Geometry check sheet. Reference: the model listing, model coordinates, mm. A direction names the side the tool comes from. Round coordinates to 2 decimals unless told otherwise and drop trailing zeros. Loops run counter-clockwise (first coordinate to the right, second up) from the corner with the lowest first, then second, coordinate; pieces in that order, holes last. Notation, with made-up numbers: (-39, -8.5) -> (16, -8.5) arc R28 cw to (16, 21.5) -> close; hole circle Ø7 at (-26, 69). An arc over 180 degrees is marked (long way). Use a Markdown table: item, result. Add a question column.
Q1. Gauge pin test, flat ends, axial feed: P1, Ø1.5, axis at x = 14.5, y = 34, coming from the -Z side; P2, Ø0.8, axis at x = 14, z = 1.5, coming from the +Y side. Record the tip position at first contact, or that the pin passes through.
Q2. Material ranges on L1, parallel to X at y = 70.5, z = 2.8 (3 decimals); L2, parallel to Z at x = 10, y = 39 (3 decimals); L3, parallel to Y at x = 93.5, z = 0.45, recorded low to high.
Q3. Release check for a two-part mould opening along X. For faces 4 (the face through (50, 39, -0.178)), 5 (the face through (101.778, 38, 2)), 6 (the face through (-0.178, 39, 2)), 7 (the face through (101.6, 39, 2)) record: released by +X, released by -X, zero draft, split by the parting line, or undercut.
Q4. Sectioned sample at C-C, the plane y = 13.5. Enter the section's corners in (x, z) (3 decimals), then the cut area to 3 significant figures.
Q5. Set-up check for faces 1 (the face through (88.9, 45, 2)), 2 (the face through (6, 76.378, 2)), 3 (the face through (12.878, 45, 2)): record each of +Z, -Z, +X, -X, +Y, -Y from which the full face is reachable in a straight line by a thin tool's end or side.
Q6. Sectioned sample at A-A, the plane y = 52. Enter the section's corners in (x, z) (3 decimals).
Q7. Sectioned sample at B-B, the plane x = 14. Enter the section's corners in (y, z) (3 decimals).
```python
from build123d import *

# Parameters (mm, degrees)
BOSS_EXTRUDE1_DEPTH = 3.175
FILLET5_R           = 1.27
SHELL2_START        = -0.1778
SHELL2_OUTLINE_W    = 75.8444
SHELL2_OUTLINE_H    = 3.5306
SHELL2_DEPTH        = 0.1778
SHELL2_START_2      = 14.942805851
SHELL2_2_OUTLINE_W  = 2.8194
SHELL2_2_OUTLINE_H  = 3.5306
SHELL2_2_DEPTH      = 0.1778
SHELL2_3_DEPTH      = 3.175
SHELL2_4_DEPTH      = 0.1778
SHELL2_START_3      = 3.175
SHELL2_5_DEPTH      = 0.1778
SHELL2_6_DEPTH      = 3.5306


with BuildPart() as part:
    # Sketch1 → Boss-Extrude1 (new body)
    with BuildSketch(Plane.XY):
        Polygon((50.8, 0), (50.8, 76.2), (15.875, 76.2), (15.875, 14.942805851), (12.7, 14.942805851), (12.7, 76.2), (0, 76.2), (0, 0), align=None)
        Polygon((85.725, 76.2), (50.8, 76.2), (50.8, 0), (101.6, 0), (101.6, 76.2), (88.9, 76.2), (88.9, 14.942805851), (85.725, 14.942805851), align=None)
    extrude(amount=BOSS_EXTRUDE1_DEPTH)

    # Fillet5
    fillet5_edges = [part.edges().sort_by_distance(p)[0] for p in [
        (0, 0, 1.5875),
        (0, 76.2, 1.5875),
        (12.7, 76.2, 1.5875),
        (15.875, 76.2, 1.5875),
        (85.725, 76.2, 1.5875),
        (88.9, 76.2, 1.5875),
        (101.6, 76.2, 1.5875),
        (101.6, 0, 1.5875),
    ]]
    fillet(fillet5_edges, radius=FILLET5_R)

    # Shell2: read off the stored shape, not the designer's step
    # Shell2 outline → Shell2 (add)
    with BuildSketch(Plane(origin=(0, 0, 0), x_dir=(1, 0, 0), z_dir=(0, 1, 0)).offset(SHELL2_START)):
        with Locations((50.8, -1.5875)):
            Rectangle(SHELL2_OUTLINE_W, SHELL2_OUTLINE_H)
    extrude(amount=SHELL2_DEPTH)

    # Shell2 2 outline → Shell2 2 (add)
    with BuildSketch(Plane(origin=(0, 0, 0), x_dir=(1, 0, 0), z_dir=(0, 1, 0)).offset(SHELL2_START_2)):
        with Locations((87.3125, -1.5875)):
            Rectangle(SHELL2_2_OUTLINE_W, SHELL2_2_OUTLINE_H)
        with Locations((14.2875, -1.5875)):
            Rectangle(SHELL2_2_OUTLINE_W, SHELL2_2_OUTLINE_H)
    extrude(amount=SHELL2_2_DEPTH)

    # Shell2 3 outline → Shell2 3 (cut)
    with BuildSketch(Plane.XY):
        with BuildLine():
            Line((1.27, 0), (100.33, 0))
            ThreePointArc((100.33, 0), (101.228025612, 0.371974388), (101.6, 1.27))
            Line((101.6, 1.27), (101.6, 74.93))
            ThreePointArc((101.6, 74.93), (101.228025612, 75.828025612), (100.33, 76.2))
            Line((100.33, 76.2), (90.17, 76.2))
            ThreePointArc((90.17, 76.2), (89.271974388, 75.828025612), (88.9, 74.93))
            Line((88.9, 74.93), (88.9, 14.942805851))
            Line((88.9, 14.942805851), (85.725, 14.942805851))
            Line((85.725, 14.942805851), (85.725, 74.93))
            ThreePointArc((85.725, 74.93), (85.353025612, 75.828025612), (84.455, 76.2))
            Line((84.455, 76.2), (17.145, 76.2))
            ThreePointArc((17.145, 76.2), (16.246974388, 75.828025612), (15.875, 74.93))
            Line((15.875, 74.93), (15.875, 14.942805851))
            Line((15.875, 14.942805851), (12.7, 14.942805851))
            Line((12.7, 14.942805851), (12.7, 74.93))
            ThreePointArc((12.7, 74.93), (12.328025612, 75.828025612), (11.43, 76.2))
            Line((11.43, 76.2), (1.27, 76.2))
            ThreePointArc((1.27, 76.2), (0.371974388, 75.828025612), (0, 74.93))
            Line((0, 74.93), (0, 1.27))
            ThreePointArc((0, 1.27), (0.371974388, 0.371974388), (1.27, 0))
        make_face()
    extrude(amount=SHELL2_3_DEPTH, mode=Mode.SUBTRACT)

    # Shell2 4 outline → Shell2 4 (add)
    with BuildSketch(Plane.XY.offset(SHELL2_START)):
        with BuildLine():
            Line((88.7222, -0.1778), (100.33, -0.1778))
            ThreePointArc((100.33, -0.1778), (101.353749198, 0.246250802), (101.7778, 1.27))
            Line((101.7778, 1.27), (101.7778, 74.93))
            ThreePointArc((101.7778, 74.93), (101.353749198, 75.953749198), (100.33, 76.3778))
            Line((100.33, 76.3778), (90.17, 76.3778))
            ThreePointArc((90.17, 76.3778), (89.146250802, 75.953749198), (88.7222, 74.93))
            Line((88.7222, 74.93), (88.7222, 14.942805851))
            Line((88.7222, 14.942805851), (85.9028, 14.942805851))
            Line((85.9028, 14.942805851), (85.9028, 74.93))
            ThreePointArc((85.9028, 74.93), (85.478749198, 75.953749198), (84.455, 76.3778))
            Line((84.455, 76.3778), (17.145, 76.3778))
            ThreePointArc((17.145, 76.3778), (16.121250802, 75.953749198), (15.6972, 74.93))
            Line((15.6972, 74.93), (15.6972, 14.942805851))
            Line((15.6972, 14.942805851), (12.8778, 14.942805851))
            Line((12.8778, 14.942805851), (12.8778, 74.93))
            ThreePointArc((12.8778, 74.93), (12.453749198, 75.953749198), (11.43, 76.3778))
            Line((11.43, 76.3778), (1.27, 76.3778))
            ThreePointArc((1.27, 76.3778), (0.246250802, 75.953749198), (-0.1778, 74.93))
            Line((-0.1778, 74.93), (-0.1778, 1.27))
            ThreePointArc((-0.1778, 1.27), (0.246250802, 0.246250802), (1.27, -0.1778))
            Line((1.27, -0.1778), (12.8778, -0.1778))
            Line((12.8778, -0.1778), (12.8778, 0))
            Line((12.8778, 0), (88.7222, 0))
            Line((88.7222, 0), (88.7222, -0.1778))
        make_face()
    extrude(amount=SHELL2_4_DEPTH)

    # Shell2 5 outline → Shell2 5 (add)
    with BuildSketch(Plane.XY.offset(SHELL2_START_3)):
        with BuildLine():
            Line((88.7222, -0.1778), (100.33, -0.1778))
            ThreePointArc((100.33, -0.1778), (101.353749198, 0.246250802), (101.7778, 1.27))
            Line((101.7778, 1.27), (101.7778, 74.93))
            ThreePointArc((101.7778, 74.93), (101.353749198, 75.953749198), (100.33, 76.3778))
            Line((100.33, 76.3778), (90.17, 76.3778))
            ThreePointArc((90.17, 76.3778), (89.146250802, 75.953749198), (88.7222, 74.93))
            Line((88.7222, 74.93), (88.7222, 14.942805851))
            Line((88.7222, 14.942805851), (85.9028, 14.942805851))
            Line((85.9028, 14.942805851), (85.9028, 74.93))
            ThreePointArc((85.9028, 74.93), (85.478749198, 75.953749198), (84.455, 76.3778))
            Line((84.455, 76.3778), (17.145, 76.3778))
            ThreePointArc((17.145, 76.3778), (16.121250802, 75.953749198), (15.6972, 74.93))
            Line((15.6972, 74.93), (15.6972, 14.942805851))
            Line((15.6972, 14.942805851), (12.8778, 14.942805851))
            Line((12.8778, 14.942805851), (12.8778, 74.93))
            ThreePointArc((12.8778, 74.93), (12.453749198, 75.953749198), (11.43, 76.3778))
            Line((11.43, 76.3778), (1.27, 76.3778))
            ThreePointArc((1.27, 76.3778), (0.246250802, 75.953749198), (-0.1778, 74.93))
            Line((-0.1778, 74.93), (-0.1778, 1.27))
            ThreePointArc((-0.1778, 1.27), (0.246250802, 0.246250802), (1.27, -0.1778))
            Line((1.27, -0.1778), (12.8778, -0.1778))
            Line((12.8778, -0.1778), (12.8778, 0))
            Line((12.8778, 0), (88.7222, 0))
            Line((88.7222, 0), (88.7222, -0.1778))
        make_face()
    extrude(amount=SHELL2_5_DEPTH)

    # Shell2 6 outline → Shell2 6 (add)
    with BuildSketch(Plane.XY.offset(SHELL2_START)):
        with BuildLine():
            Line((88.7222, -0.1778), (100.33, -0.1778))
            ThreePointArc((100.33, -0.1778), (101.353749198, 0.246250802), (101.7778, 1.27))
            Line((101.7778, 1.27), (101.7778, 74.93))
            ThreePointArc((101.7778, 74.93), (101.353749198, 75.953749198), (100.33, 76.3778))
            Line((100.33, 76.3778), (90.17, 76.3778))
            ThreePointArc((90.17, 76.3778), (89.146250802, 75.953749198), (88.7222, 74.93))
            Line((88.7222, 74.93), (88.7222, 14.942805851))
            Line((88.7222, 14.942805851), (88.9, 14.942805851))
            Line((88.9, 14.942805851), (88.9, 74.93))
            ThreePointArc((88.9, 74.93), (89.271974388, 75.828025612), (90.17, 76.2))
            Line((90.17, 76.2), (100.33, 76.2))
            ThreePointArc((100.33, 76.2), (101.228025612, 75.828025612), (101.6, 74.93))
            Line((101.6, 74.93), (101.6, 1.27))
            ThreePointArc((101.6, 1.27), (101.228025612, 0.371974388), (100.33, 0))
            Line((100.33, 0), (88.7222, 0))
            Line((88.7222, 0), (88.7222, -0.1778))
        make_face()
        with BuildLine():
            Line((1.27, -0.1778), (12.8778, -0.1778))
            Line((12.8778, -0.1778), (12.8778, 0))
            Line((12.8778, 0), (1.27, 0))
            ThreePointArc((1.27, 0), (0.371974388, 0.371974388), (0, 1.27))
            Line((0, 1.27), (0, 74.93))
            ThreePointArc((0, 74.93), (0.371974388, 75.828025612), (1.27, 76.2))
            Line((1.27, 76.2), (11.43, 76.2))
            ThreePointArc((11.43, 76.2), (12.328025612, 75.828025612), (12.7, 74.93))
            Line((12.7, 74.93), (12.7, 14.942805851))
            Line((12.7, 14.942805851), (12.8778, 14.942805851))
            Line((12.8778, 14.942805851), (12.8778, 74.93))
            ThreePointArc((12.8778, 74.93), (12.453749198, 75.953749198), (11.43, 76.3778))
            Line((11.43, 76.3778), (1.27, 76.3778))
            ThreePointArc((1.27, 76.3778), (0.246250802, 75.953749198), (-0.1778, 74.93))
            Line((-0.1778, 74.93), (-0.1778, 1.27))
            ThreePointArc((-0.1778, 1.27), (0.246250802, 0.246250802), (1.27, -0.1778))
        make_face()
        with BuildLine():
            Line((85.725, 14.942805851), (85.9028, 14.942805851))
            Line((85.9028, 14.942805851), (85.9028, 74.93))
            ThreePointArc((85.9028, 74.93), (85.478749198, 75.953749198), (84.455, 76.3778))
            Line((84.455, 76.3778), (17.145, 76.3778))
            ThreePointArc((17.145, 76.3778), (16.121250802, 75.953749198), (15.6972, 74.93))
            Line((15.6972, 74.93), (15.6972, 14.942805851))
            Line((15.6972, 14.942805851), (15.875, 14.942805851))
            Line((15.875, 14.942805851), (15.875, 74.93))
            ThreePointArc((15.875, 74.93), (16.246974388, 75.828025612), (17.145, 76.2))
            Line((17.145, 76.2), (84.455, 76.2))
            ThreePointArc((84.455, 76.2), (85.353025612, 75.828025612), (85.725, 74.93))
            Line((85.725, 74.93), (85.725, 14.942805851))
        make_face()
    extrude(amount=SHELL2_6_DEPTH)


solid = part.part
```
Values:
| question | item | result |
|---|---|---|
| 1 | P1 | through |
| 1 | P2 | y = 15.12 |
| 2 | L1 | -0.178 to 0, 12.7 to 12.878, 15.697 to 15.875, 85.725 to 85.903, 88.722 to 88.9, 101.6 to 101.778 |
| 2 | L2 | -0.178 to 0, 3.175 to 3.353 |
| 2 | L3 | -0.18 to 0, 76.2 to 76.38 |
| 3 | face 4 | zero draft |
| 3 | face 5 | released by +X |
| 3 | face 6 | released by -X |
| 3 | face 7 | undercut |
| 4 | outline | (-0.178, -0.178) -> (101.778, -0.178) -> (101.778, 3.353) -> (-0.178, 3.353) -> close; hole (0, 0) -> (101.6, 0) -> (101.6, 3.175) -> (0, 3.175) -> close |
| 4 | area | 37.4 mm^2 |
| 5 | face 1 | none |
| 5 | face 2 | +Z, -Z, +X, -X, +Y |
| 5 | face 3 | +Z, -Z, +Y |
| 6 | outline | (-0.178, -0.178) -> (12.878, -0.178) -> (12.878, 3.353) -> (-0.178, 3.353) -> close; (15.697, -0.178) -> (85.903, -0.178) -> (85.903, 3.353) -> (15.697, 3.353) -> close; (88.722, -0.178) -> (101.778, -0.178) -> (101.778, 3.353) -> (88.722, 3.353) -> close; hole (0, 0) -> (12.7, 0) -> (12.7, 3.175) -> (0, 3.175) -> close; hole (15.875, 0) -> (85.725, 0) -> (85.725, 3.175) -> (15.875, 3.175) -> close; hole (88.9, 0) -> (101.6, 0) -> (101.6, 3.175) -> (88.9, 3.175) -> close |
| 7 | outline | (-0.178, -0.178) -> (15.121, -0.178) -> (15.121, 3.353) -> (-0.178, 3.353) -> close; hole (0, 0) -> (14.943, 0) -> (14.943, 3.175) -> (0, 3.175) -> close |
